Part model, mm, in its own coordinate system. Give positions to 0.01 mm unless a question says otherwise; leave off trailing zeros. Write each loop counter-clockwise with the first axis right and the second up, starting at its lowest first coordinate (ties: lowest second). Pieces come first, ordered by that corner, then holes.
```python
from build123d import *

# Parameters (mm, degrees)
SKETCH1_R           = 20
BOSS_EXTRUDE1_DEPTH = 30
BOSS_EXTRUDE1_DRAFT = -10
SKETCH5_R           = 28
BOSS_EXTRUDE3_DEPTH = 15
BOSS_EXTRUDE3_DRAFT = -10
SKETCH6_R           = 24
CUT_EXTRUDE3_DEPTH  = 40
CUT_EXTRUDE3_DRAFT  = -10
CUT_EXTRUDE4_REACH  = 60.976
SKETCH7_R           = 4


with BuildPart() as part:
    # Sketch1 → Boss-Extrude1 (with draft: the straight prism first)
    with BuildSketch(Plane(origin=(0, 0, 0), x_dir=(1, 0, 0), z_dir=(0, 1, 0))):
        Circle(SKETCH1_R)
    extrude(amount=BOSS_EXTRUDE1_DEPTH)
    # Boss-Extrude1: the draft: its side faces are tilted about the plane it starts from
    boss_extrude1_sides = [part.faces().sort_by_distance(p)[0] for p in [
        (-20, 15, 0),
    ]]
    draft(boss_extrude1_sides, Plane(origin=(0, 0, 0), x_dir=(1, 0, 0), z_dir=(0, 1, 0)), BOSS_EXTRUDE1_DRAFT)


with BuildPart() as boss_extrude3_tool:
    # Sketch5 → Boss-Extrude3 (with draft: the straight prism first)
    with BuildSketch(Plane(origin=(0, 30, 0), x_dir=(1, 0, 0), z_dir=(0, 1, 0))):
        Circle(SKETCH5_R)
    extrude(amount=BOSS_EXTRUDE3_DEPTH)
    # Boss-Extrude3: the draft: its side faces are tilted about the plane it starts from
    boss_extrude3_sides = [boss_extrude3_tool.faces().sort_by_distance(p)[0] for p in [
        (-28, 37.5, 0),
    ]]
    draft(boss_extrude3_sides, Plane(origin=(0, 30, 0), x_dir=(1, 0, 0), z_dir=(0, 1, 0)), BOSS_EXTRUDE3_DRAFT)


with BuildPart() as part_1:
    add(part.part)

    # Boss-Extrude3: add boss_extrude3_tool
    add(boss_extrude3_tool.part)


with BuildPart() as cut_extrude3_tool:
    # Sketch6 → Cut-Extrude3 (with draft: the straight prism first)
    with BuildSketch(Plane(origin=(0, 45, 0), x_dir=(1, 0, 0), z_dir=(0, 1, 0))):
        Circle(SKETCH6_R)
    extrude(amount=-CUT_EXTRUDE3_DEPTH)
    # Cut-Extrude3: the draft: its side faces are tilted about the plane it starts from
    cut_extrude3_sides = [cut_extrude3_tool.faces().sort_by_distance(p)[0] for p in [
        (-24, 25, 0),
    ]]
    draft(cut_extrude3_sides, Plane(origin=(0, 45, 0), x_dir=(1, 0, 0), z_dir=(0, 1, 0)), CUT_EXTRUDE3_DRAFT)


with BuildPart() as part_2:
    add(part_1.part)

    # Cut-Extrude3: cut by cut_extrude3_tool
    add(cut_extrude3_tool.part, mode=Mode.SUBTRACT)

    # Sketch7 → Cut-Extrude4 (cut, up to next)
    with BuildSketch(Plane(origin=(0, 5, 0), x_dir=(1, 0, 0), z_dir=(0, 1, 0)), mode=Mode.PRIVATE) as cut_extrude4_sk1:
        with Locations(Location((0, 0, 0), (0, 0, 270))):
            Circle(SKETCH7_R)
    cut_extrude4_tool1 = extrude(cut_extrude4_sk1.sketch, amount=-CUT_EXTRUDE4_REACH, mode=Mode.PRIVATE) & part_2.part
    add(cut_extrude4_tool1.solids().sort_by_distance((0, 5, 0))[0], mode=Mode.SUBTRACT)


solid = part_2.part
```
1) Saw through at D-D, the plane y = 33. Write the cut outline in (x, z), then the cut area to 3 significant figures.
Answers follow:
outline: circle Ø57.06 at (0, 0); hole circle Ø43.77 at (0, 0)
area: 1,050 mm2
2) Saw through at A-A, the plane z = 0. Write the cut outline in (x, y), then the cut area to 3 significant figures.
Answers follow:
outline: (-30.64, 45) - (-28, 30) - (-25.29, 30) - (-20, 0) - (-4, 0) - (-4, 5) - (-16.95, 5) - (-24, 45) - close; (4, 0) - (20, 0) - (25.29, 30) - (28, 30) - (30.64, 45) - (24, 45) - (16.95, 5) - (4, 5) - close
area: 560 mm2
3) Saw through at C-C, the plane y = 12.5. Write the cut outline in (x, z), then the cut area to 3 significant figures.
Answers follow:
outline: circle Ø44.41 at (0, 0); hole circle Ø36.54 at (0, 0)
area: 500 mm2
4) Pin check, flat tips, straight feed: pin 1 Ø4 at (x, z) = (24.5, -16) entering from -Y; pin 2 Ø4 at (y, z) = (5.5, 12) entering from +X; pin 3 Ø6 at (x, y) = (22.5, 33.5) entering from +Z; pin 4 Ø7 at (x, z) = (0, 0) entering from -Y. Stop position of each tip, or through.
Answers follow:
pin 1: stops at y = 30
pin 2: stops at x = 18.5
pin 3: stops at z = 21.04
pin 4: passes through
5) Wall check: L1, parallel to Y at x = -11.5, z = -8.5; L2, parallel to Y at x = 13, z = -22; L3, parallel to X at y = 1.7, z = 0. Give the ranges that are in metal, low to high.
Answers follow:
L1: y = 0 to 5
L2: y = 30 to 45
L3: x = -20.3 to -4, 4 to 20.3
6) Saw through at B-B, the plane x = 0. Write the cut outline in (y, z).
Answers follow:
outline: (0, -20) - (30, -25.29) - (30, -28) - (45, -30.64) - (45, -24) - (5, -16.95) - (5, -4) - (0, -4) - close; (0, 4) - (5, 4) - (5, 16.95) - (45, 24) - (45, 30.64) - (30, 28) - (30, 25.29) - (0, 20) - close
7) Two-plate mould, pull along X, no slides. Class faces 1 (the face through (-3.905, 2.535, -0.867)), 2 (the face through (-6, 30, 25)), 3 (the face through (20.341, 11.457, 8.434)), 4 (the face through (4, 5, 4)): +X half, -X half, draft (parallel to the pull), parting line (faces both ways), or undercut.
Answers follow:
face 1: undercut
face 2: draft
face 3: parting line
face 4: undercut
